from build123d import *

# Parameters (mm, degrees)
F0_W     = 40
F0_H     = 40
F0_R     = 1.5
F1_DEPTH = 10
F3_DEPTH = 7
F4_R     = 3
F5_DEPTH = 3
F6_R     = 1.5
F7_DEPTH = 3.001


with BuildPart() as f1:
    # F0 (on Top) → F1 (new body)
    with BuildSketch(Plane.XY):
        Rectangle(F0_W, F0_H)
        with Locations((0, -16)):
            Circle(F0_R, mode=Mode.SUBTRACT)
        with Locations((-16, 0)):
            Circle(F0_R, mode=Mode.SUBTRACT)
        with Locations((16, 0)):
            Circle(F0_R, mode=Mode.SUBTRACT)
        with Locations((0, 16)):
            Circle(F0_R, mode=Mode.SUBTRACT)
    extrude(amount=F1_DEPTH)

    # F2 (on face) → F3 (cut)
    with BuildSketch(Plane.XY.offset(10)):
        with BuildLine():
            Line((7, 12), (-7, 12))
            ThreePointArc((-7, 12), (-15.535534, 15.535534), (-12, 7))
            Line((-12, 7), (-12, -7))
            ThreePointArc((-12, -7), (-15.535534, -15.535534), (-7, -12))
            Line((-7, -12), (7, -12))
            ThreePointArc((7, -12), (15.535534, -15.535534), (12, -7))
            Line((12, -7), (12, 7))
            ThreePointArc((12, 7), (15.535534, 15.535534), (7, 12))
        make_face()
    extrude(amount=-F3_DEPTH, mode=Mode.SUBTRACT)

    # F4 (on face) → F5 (cut)
    with BuildSketch(Plane(origin=(0, 0, 0), x_dir=(1, 0, 0), z_dir=(0, 0, -1))):
        with Locations((0, 16)):
            Circle(F4_R)
        with Locations((-16, 0)):
            Circle(F4_R)
        with Locations((0, -16)):
            Circle(F4_R)
        with Locations((16, 0)):
            Circle(F4_R)
    extrude(amount=-F5_DEPTH, mode=Mode.SUBTRACT)

    # F6 (on face) → F7 (cut, through all)
    with BuildSketch(Plane.XY.offset(3)):
        with Locations((-8.5, 8.5)):
            Circle(F6_R)
        with Locations((8.5, 8.5)):
            Circle(F6_R)
        with Locations((-8.5, -8.5)):
            Circle(F6_R)
        with Locations((8.5, -8.5)):
            Circle(F6_R)
    extrude(amount=-F7_DEPTH, mode=Mode.SUBTRACT)


solid = f1.part
Could you check a few things on this model? Use its own coordinates, in mm. A direction names the side the tool comes from. Give positions to 0.01 mm unless a question says otherwise; leave off trailing zeros. Loops run counter-clockwise (first coordinate to the right, second up) from the corner with the lowest first, then second, coordinate; pieces in that order, holes last. Notation, with made-up numbers: (22, -23.5) -> (73, -23.5) arc R25 cw to (73, -2.5) -> close; hole circle Ø5 at (-25.5, 64). An arc over 180 degrees is marked (long way). Answer as CSV lines item,"result". Start each with the question number.
(1) If we section it at B-B on x = -16: Write out the boundary of the cut face in (y, z), then the cut area to 3 significant figures.
(2) I'm going to push flat-ended pins straight in: pin 1 Ø9 at (x, y) = (12, -12) entering from +Z; pin 2 Ø5 at (x, y) = (-16, 0) entering from -Z. Where does each tip first touch, or does it pass through?
(3) We'd pull the mould along X, two halves only. Please class faces 4 (the flat face through (0, 0, 0)), 5 (the cylindrical face through (16, 15, 7)): released by +X, released by -X, zero draft, split by the parting line, or undercut.
(4) Which directions (+Z, -Z, +X, -X, +Y, -Y) give clear straight access to the entire face, cutting with the end or side of a thin tool? Please do faces 1 (the cylindrical face through (-19, 0, 1)), 2 (the cylindrical face through (7.3, -9.4, 1.5)), 3 (the cylindrical face through (-16, -15, 7)).
(5) I need wall thicknesses on probe 1 along Y at (x, z) = (0, 8); probe 2 along Y at (x, z) = (-8.5, 0.85). Which ranges of each line are inside material? Lowest first, please.
(6) If we section it at D-D on y = 8.5: Write out the boundary of the cut face in (x, z).
(7) If we section it at A-A on z = 6: Write out the boundary of the cut face in (x, y), then the cut area to 3 significant figures.
Computed:
1,outline,"(-20, 0) -> (-3, 0) -> (-3, 3) -> (-1.5, 3) -> (-1.5, 10) -> (-9, 10) -> (-9, 3) -> (-15, 3) -> (-15, 10) -> (-20, 10) -> close; (1.5, 3) -> (3, 3) -> (3, 0) -> (20, 0) -> (20, 10) -> (15, 10) -> (15, 3) -> (9, 3) -> (9, 10) -> (1.5, 10) -> close"
1,area,"277 mm2"
2,pin 1,"stops at z = 3"
2,pin 2,"stops at z = 3"
3,face 4,"zero draft"
3,face 5,"undercut"
4,face 1,"-Z"
4,face 2,"+Z, -Z"
4,face 3,"+Z"
5,probe 1,"y = -20 to -17.5, -14.5 to -12, 12 to 14.5, 17.5 to 20"
5,probe 2,"y = -20 to -10, -7 to 7, 10 to 20"
6,outline,"(-20, 0) -> (-10, 0) -> (-10, 3) -> (-15.57, 3) -> (-15.57, 10) -> (-20, 10) -> close; (-7, 0) -> (7, 0) -> (7, 3) -> (-7, 3) -> close; (10, 0) -> (20, 0) -> (20, 10) -> (15.57, 10) -> (15.57, 3) -> (10, 3) -> close"
7,outline,"(-20, -20) -> (20, -20) -> (20, 20) -> (-20, 20) -> close; hole circle Ø3 at (-16, 0); hole (-12, -7) arc R5 ccw (long way) to (-7, -12) -> (7, -12) arc R5 ccw (long way) to (12, -7) -> (12, 7) arc R5 ccw (long way) to (7, 12) -> (-7, 12) arc R5 ccw (long way) to (-12, 7) -> close; hole circle Ø3 at (0, -16); hole circle Ø3 at (0, 16); hole circle Ø3 at (16, 0)"
7,area,"760 mm2"
